```python
from build123d import *

# Parameters (mm, degrees)
PAD_DEPTH       = 7.5
POCKET_DEPTH    = 4.5
SKETCH002_R     = 3
POCKET001_DEPTH = 5.001


with BuildPart() as part:
    # Sketch → Pad (new body, symmetric)
    with BuildSketch(Plane.XY):
        Polygon((7.25, 5), (7.25, 2.1), (4.641857, 0), (0, 0), (-4.641857, 0), (-7.25, 2.1), (-7.25, 5), (0, 5), align=None)
    extrude(amount=PAD_DEPTH, both=True)

    # Sketch001 (on Face1 of Pad) → Pocket (cut)
    with BuildSketch(Plane(origin=(0, 5, 0), x_dir=(-1, 0, 0), z_dir=(0, 1, 0))):
        Polygon((0, 5.91784), (-5.125, 2.95892), (-5.125, -2.95892), (0, -5.91784), (5.125, -2.95892), (5.125, 2.95892), align=None)
    extrude(amount=-POCKET_DEPTH, mode=Mode.SUBTRACT)

    # Sketch002 (on Face1 of Pocket) → Pocket001 (cut, through all)
    with BuildSketch(Plane(origin=(0, 5, 0), x_dir=(-1, 0, 0), z_dir=(0, 1, 0))):
        Circle(SKETCH002_R)
    extrude(amount=-POCKET001_DEPTH, mode=Mode.SUBTRACT)


solid = part.part
```
Input: part model. Units: mm. Frame: model coordinates. A direction names the side the tool comes from. Give positions to 0.01 mm unless a question says otherwise; leave off trailing zeros. Order: outer loops, then holes, each group sorted by start corner. A loop starts at its lowest first (then second) coordinate and runs counter-clockwise, first axis right, second up. Notation, with made-up numbers: (-27, 69.25) - (-17, 69.25) arc R22 ccw to (-17, 108.25) - close; hole circle Ø1 at (-21, 34.5). An arc over 180 degrees is marked (long way). One line per item, written item: value.
1. Line query: probe 1 along Z at (x, y) = (0, 0.35); probe 2 along X at (y, z) = (3.9, 2.25) (3 decimals); probe 3 along Y at (x, z) = (-2.75, 3). Output: solid intervals per line, ascending.
Determined:
probe 1: -7.5 to -3, 3 to 7.5
probe 2: -7.25 to -5.125, 5.125 to 7.25
probe 3: 0 to 0.5
2. Pin query (flat end, axial travel): pin 1 Ø6 at (x, z) = (0.5, 0.5) entering from +Y; pin 2 Ø3 at (x, z) = (-0.5, 1) entering from +Y. Return the tip coordinate at first contact, or that it passes through.
Determined:
pin 1: y = 0.5
pin 2: through
3. Cut plane C-C, the plane x = 1.25. Output: boundary loops of the cut face in (y, z).
Determined:
outline: (0, -7.5) - (5, -7.5) - (5, -5.2) - (0.5, -5.2) - (0.5, -2.73) - (0, -2.73) - close; (0, 2.73) - (0.5, 2.73) - (0.5, 5.2) - (5, 5.2) - (5, 7.5) - (0, 7.5) - close
4. Cut plane D-D, the plane y = 1.45. Output: boundary loops of the cut face in (x, z) (3 decimals), and give its area (3 significant figures).
Determined:
outline: (-6.443, -7.5) - (6.443, -7.5) - (6.443, 7.5) - (-6.443, 7.5) - close; hole (-5.125, -2.959) - (0, -5.918) - (5.125, -2.959) - (5.125, 2.959) - (0, 5.918) - (-5.125, 2.959) - close
area: 102 mm2
5. Cut plane A-A, the plane z = 0. Output: boundary loops of the cut face in (x, y) (3 decimals), and give its area (3 significant figures).
Determined:
outline: (-7.25, 2.1) - (-4.642, 0) - (-3, 0) - (-3, 0.5) - (-5.125, 0.5) - (-5.125, 5) - (-7.25, 5) - close; (3, 0) - (4.642, 0) - (7.25, 2.1) - (7.25, 5) - (5.125, 5) - (5.125, 0.5) - (3, 0.5) - close
area: 17.9 mm2
6. Draft query along Z for faces 1 (the face through (2.527, 2.782, 4.459)), 2 (the face through (0, 3, 7.5)), 3 (the face through (-5.928, 1.035, 0.105)), 4 (the face through (5.125, 3, 0)). Return one class per face: released by +Z, released by -Z, zero draft, split by the parting line, or undercut.
Determined:
face 1: undercut
face 2: released by +Z
face 3: zero draft
face 4: undercut
7. Reachability of faces 5 (the face through (-3.2, 0, 0.1)), 6 (the face through (2, 0.5, -3)) from +Z, -Z, +X, -X, +Y, -Y: full face, straight path, thin tool, end or side. Return the list, or none.
Determined:
face 5: +Z, -Z, +X, -X, -Y
face 6: +Y
8. Cut plane B-B, the plane y = 3. Output: boundary loops of the cut face in (x, z) (3 decimals).
Determined:
outline: (-7.25, -7.5) - (7.25, -7.5) - (7.25, 7.5) - (-7.25, 7.5) - close; hole (-5.125, -2.959) - (0, -5.918) - (5.125, -2.959) - (5.125, 2.959) - (0, 5.918) - (-5.125, 2.959) - close
